Geometry check sheet. Reference: the model listing, model coordinates, mm. A direction names the side the tool comes from. Give positions to 0.01 mm unless a question says otherwise; leave off trailing zeros. Write each loop counter-clockwise with the first axis right and the second up, starting at its lowest first coordinate (ties: lowest second). Pieces come first, ordered by that corner, then holes.
(1) Tool access check on faces 1 (the cylindrical face through (31.75, 50.92, 1.61)), 2 (the flat face through (-5.85, 61.16, 1.57)). Record the directions out of +Z, -Z, +X, -X, +Y, -Y that give a thin tool (end or side, any length) a straight path to the whole face; none if there is none.
(2) Cross-section at D-D (z = 1.3). Record the boundary of the cut face in (x, y).
(3) Thickness scan on line 1 along Y through (x, z) = (26, 0.55); line 2 along X through (y, z) = (51, 1.05); line 3 along X through (y, z) = (47, 2.35). Record the ranges inside material, lowest first.
(4) Cross-section at B-B (x = 12.7). Record the boundary of the cut face in (y, z) (3 decimals), and give its area (3 significant figures).
(5) Cross-section at A-A (y = 31.75). Record the boundary of the cut face in (x, z) (3 decimals).
(6) Cross-section at C-C (x = 76.2). Record the boundary of the cut face in (y, z) (3 decimals).
(7) Mould release check, pull along Y, two halves, no side actions. Record for faces 3 (the flat face through (-6.144, 4.915, 1.565)), 4 (the cylindrical face through (60.287, 48.141, 1.565)), 5 (the cylindrical face through (100.836, 62.776, 1.61)): +Y half, -Y half, draft (parallel to the pull), parting line (faces both ways), or undercut.
(8) Depth check by flat-ended pin: P1, Ø6, axis at x = 12.7, y = 12.7, coming from the +Z side. Enter the tip coordinate at first touch or a pass-through.
```python
from build123d import *

# Parameters (mm, degrees)
BOSS_EXTRUDE1_DEPTH              = 3.175
SKETCH2_R                        = 19.177
CUT_EXTRUDE1_DEPTH               = 3.175
SKETCH3_R                        = 3.3734375
CUT_EXTRUDE2_DEPTH               = 3.175
CUT_EXTRUDE3_DEPTH               = 120.85362166
FILLET1_R                        = 2.54
F_13_64_0_20313_DIAMETER_HOLE1_D = 5.159502


with BuildPart() as part:
    # Sketch1 → Boss-Extrude1 (new body)
    with BuildSketch(Plane.XY):
        Polygon((-12.7, 58.42), (0, 63.5), (101.6, 63.5), (101.6, 0), (0, 0), (-12.7, 10.16), align=None)
    extrude(amount=BOSS_EXTRUDE1_DEPTH)

    # Sketch2 → Cut-Extrude1 (cut)
    with BuildSketch(Plane.XY.offset(3.175)):
        with Locations((76.2, 31.75)):
            Circle(SKETCH2_R)
    extrude(amount=-CUT_EXTRUDE1_DEPTH, mode=Mode.SUBTRACT)

    # Sketch3 → Cut-Extrude2 (cut)
    with BuildSketch(Plane.XY.offset(3.175)):
        with Locations((12.7, 12.7)):
            Circle(SKETCH3_R)
    extrude(amount=-CUT_EXTRUDE2_DEPTH, mode=Mode.SUBTRACT)

    # Sketch4 → Cut-Extrude3 (cut, through all)
    with BuildSketch(Plane.XY.offset(3.175)):
        with BuildLine():
            Line((-0.79375, 56.35625), (26.19375, 56.35625))
            ThreePointArc((26.19375, 56.35625), (31.75, 50.8), (26.19375, 45.24375))
            Line((26.19375, 45.24375), (-0.79375, 45.24375))
            ThreePointArc((-0.79375, 45.24375), (-6.35, 50.8), (-0.79375, 56.35625))
        make_face()
    extrude(amount=-CUT_EXTRUDE3_DEPTH, mode=Mode.SUBTRACT)

    # Fillet1
    fillet1_edges = [part.edges().sort_by_distance(p)[0] for p in [
        (-12.7, 10.16, 1.5875),
        (-12.7, 58.42, 1.5875),
        (0, 63.5, 1.5875),
        (101.6, 63.5, 1.5875),
        (101.6, 0, 1.5875),
        (0, 0, 1.5875),
    ]]
    fillet(fillet1_edges, radius=FILLET1_R)

    # 13/64 (0.20313) Diameter Hole1 (through all)
    with Locations(Plane.XY.offset(3.175)):
        with Locations((58.239487758, 49.710512242), (94.160512242, 49.710512242), (94.160512242, 13.789487758), (58.239487758, 13.789487758)):
            Hole(F_13_64_0_20313_DIAMETER_HOLE1_D / 2)


solid = part.part
```
Reply:
1. face 1: +Z, -Z
1. face 2: +Z, -Z, -X, +Y
2. outline: (-12.7, 11.38) arc R2.54 ccw to (-11.75, 9.4) - (-0.7, 0.56) arc R2.54 ccw to (0.89, 0) - (99.06, 0) arc R2.54 ccw to (101.6, 2.54) - (101.6, 60.96) arc R2.54 ccw to (99.06, 63.5) - (0.49, 63.5) arc R2.54 ccw to (-0.45, 63.32) - (-11.1, 59.06) arc R2.54 ccw to (-12.7, 56.7) - close; hole (-0.79, 45.24) - (26.19, 45.24) arc R5.56 ccw to (26.19, 56.36) - (-0.79, 56.36) arc R5.56 ccw to start; hole circle Ø6.75 at (12.7, 12.7); hole circle Ø5.16 at (58.24, 13.79); hole circle Ø5.16 at (58.24, 49.71); hole circle Ø38.35 at (76.2, 31.75); hole circle Ø5.16 at (94.16, 13.79); hole circle Ø5.16 at (94.16, 49.71)
3. line 1: y = 0 to 45.24, 56.36 to 63.5
3. line 2: x = -12.7 to -6.35, 31.75 to 56.01, 60.47 to 91.93, 96.39 to 101.6
3. line 3: x = -12.7 to -4.85, 30.25 to 64.57, 87.83 to 101.6
4. outline: (0, 0) - (9.327, 0) - (9.327, 3.175) - (0, 3.175) - close; (16.073, 0) - (45.244, 0) - (45.244, 3.175) - (16.073, 3.175) - close; (56.356, 0) - (63.5, 0) - (63.5, 3.175) - (56.356, 3.175) - close
4. area: 145 mm2
5. outline: (-12.7, 0) - (57.023, 0) - (57.023, 3.175) - (-12.7, 3.175) - close; (95.377, 0) - (101.6, 0) - (101.6, 3.175) - (95.377, 3.175) - close
6. outline: (0, 0) - (12.573, 0) - (12.573, 3.175) - (0, 3.175) - close; (50.927, 0) - (63.5, 0) - (63.5, 3.175) - (50.927, 3.175) - close
7. face 3: -Y half
7. face 4: undercut
7. face 5: +Y half
8. P1: passes through
